Here's how the part is built. I have some questions about the finished solid (model axes, mm). Coordinates: 2 decimals unless noted, no trailing zeros. Write each loop counter-clockwise with the first axis right and the second up, starting at its lowest first coordinate (ties: lowest second). Pieces come first, ordered by that corner, then holes.
Item 1: If we section it at A-A (y = 0): Please give me the cut outline in (x, z).
Item 2: We'd pull the mould along Z, two halves only. Please class faces 1 (the face through (4.93, -9.902, -49.786)), 2 (the face through (5, 5, -42)), 3 (the face through (5, -57, -82)), 4 (the face through (4.93, -37.92, -66.82)): +Z half, -Z half, draft (parallel to the pull), parting line (faces both ways), or undercut.
Item 3: I'm going to push a flat-ended pin straight in: pin 1 Ø5 at (y, z) = (-9.58, -66.75) entering from +X. Where does the tip first touch, or does it pass through?
Item 4: If we section it at B-B (z = -23): Please give me the cut outline in (x, y), then the cut area to 3 significant figures.
Item 5: If we section it at C-C (z = -39): Please give me the cut outline in (x, y), then the cut area to 3 significant figures.
Item 6: If we section it at D-D (y = -16.5): Please give me the cut outline in (x, z).
Item 7: If I drill on line 1 (Z direction, x = 5.5, y = -23); line 2 (Y direction, x = 5, z = -66.75); line 3 (Z direction, x = 6.5, y = -30), over which ranges is the centre line in solid material (lowest first)?
Autodesk Inventor part; units mm, degrees
ref_plane "YZ Plane" through (0, 0, 0) normal (1, 0, 0) x (0, 1, 0)
ref_plane "XZ Plane" through (0, 0, 0) normal (0, 1, 0) x (-1, 0, 0)
ref_plane "XY Plane" through (0, 0, 0) normal (0, 0, 1) x (1, 0, 0)
sketch "Esquisse1" plane through (0, 0, 0) normal (1, 0, 0) x (0, 1, 0)
  line L0 (0, 0) -> (-126, 0)
  line L1 (-126, -82) -> (0, -82)
  circle A0 centre (-23, -23) radius 18
  circle A1 centre (-23, -59) radius 18
  circle A2 centre (-116.2792, -41) radius 4
  line L2 (-120.2792, 0) -> (-120.2792, -82)
  circle A3 centre (-30, -59) radius 6
  circle A4 centre (-23, -43.5) radius 1.5
  circle A5 centre (-23, -74.5) radius 1.5
  circle A6 centre (-9.5766, -51.25) radius 1.5
  circle A7 centre (-9.5766, -66.75) radius 1.5
  line L3 (-23, -59) -> (-30, -59)
  line L4 (-23, -59) -> (-23, -43.5)
  line L5 (-23, -59) -> (-23, -74.5)
  circle A8 centre (-36.4234, -51.25) radius 1.5
  circle A9 centre (-36.4234, -66.75) radius 1.5
  line L6 (0, -82) -> (5, -82)
  line L7 (5, -82) -> (5, 0)
  line L8 (5, 0) -> (0, 0)
  line L9 (-5, -82) -> (-5, 0)
  line L10 (0, -72) -> (0, -10)
  circle A10 centre (0, -72) radius 2
  circle A11 centre (0, -10) radius 2
  line L11 (5, 0) -> (0, 0)
  line L12 (5, -82) -> (-5, -82)
  line L13 (-107.2792, -10) -> (-107.2792, -72)
  circle A12 centre (-107.2792, -10) radius 2
  circle A13 centre (-107.2792, -72) radius 2
  line L14 (-120.2792, 0) -> (-126, 0)
  line L15 (-126, 0) -> (-126, -82)
  line L16 (-126, -82) -> (-120.2792, -82)
  line L17 (-120.2792, -82) -> (-120.2792, 0)
  dimension "d0" = 82
  dimension "d2" = 36
  dimension "d3" = 23
  dimension "d4" = 36
  dimension "d5" = 23
  dimension "d6" = 8
  dimension "d7" = 95
  dimension "d8" = 41
  dimension "d12" = 4
  dimension "d13" = 12
  dimension "d14" = 7
  dimension "d15" = 3
  dimension "d16" = 15.5
  dimension "d17" = 3
  dimension "d18" = 15.5
  dimension "d19" = 3
  dimension "d20" = 3
  dimension "d21" = 60
  dimension "d22" = 60
  dimension "d23" = 15.5
  dimension "d25" = 0
  dimension "d26" = 15.5
  dimension "d27" = 3
  dimension "d28" = 3
  dimension "d29" = 15.5
  dimension "d30" = 15.5
  dimension "d31" = 60
  dimension "d32" = 60
  dimension "d38" = 82
  dimension "d39" = 28
  dimension "d40" = 10
  dimension "d41" = 5
  dimension "d42" = 62
  dimension "d43" = 10
  dimension "d44" = 4
  dimension "d45" = 4
  dimension "d46" = 5
  dimension "d47" = 82
  dimension "d48" = 10
  dimension "d49" = 28
  dimension "d61" = 62
  dimension "d62" = 13
  dimension "d63" = 10
  dimension "d64" = 4
  dimension "d65" = 4
  dimension "d76" = 126
  dimension "d77" = 126
extrude "Extrusion1" add sketch "Esquisse1" along normal blind 10 contours L9 A0 A1 L1 L2 L0 | L9 A1 A0 | A1 | A13 | A12
sketch "Esquisse2" plane through (10, -23, -23) normal (1, 0, 0) x (0, 0, -1)
  line L0 (0, 18) -> (-23, 18)
  line L1 (-23, 18) -> (59, 18)
  line L2 (59, 18) -> (59, 28)
  line L3 (59, 28) -> (-23, 28)
  line L4 (-23, 28) -> (-23, 18)
  line L5 (-13, 23) -> (49, 23)
  circle A0 centre (-13, 23) radius 2
  circle A1 centre (49, 23) radius 2
  point P0 (-23, 23)
  dimension "d52" = 82
  dimension "d53" = 10
  dimension "d54" = 62
  dimension "d55" = 10
  dimension "d56" = 4
  dimension "d57" = 4
  dimension "d58" = 5
extrude "Extrusion2" add sketch "Esquisse2" against normal blind 10
sketch "Esquisse3" plane through (10, -116.2792, -41) normal (1, 0, 0) x (0, 0, -1)
  line L0 (-31, 9) -> (31, 9)
  line L1 (-41, 121.2792) -> (-41, -4)
  line L2 (-41, -4) -> (0, -4)
  point P0 (-41, 116.2792)
  dimension "d66" = 62
  dimension "d67" = 10
  dimension "d68" = 13
hole "Perçage1" at (10, -107.2792, -10) at (10, -107.2792, -72) direction (-1, 0, 0) diameter 4 end through all
sketch "Esquisse4" plane through (0, -120.2792, -41) normal (0, -1, 0) x (1, 0, 0)
  line L0 (0, 0) -> (0, -41)
  line L1 (10, 41) -> (0, 41)
  line L2 (0, 41) -> (0, -41)
  line L3 (0, -41) -> (10, -41)
  line L4 (10, -41) -> (10, 41)
  dimension "d78" = 10
  dimension "d79" = 82
extrude "Extrusion3" add sketch "Esquisse4" along normal blind 0.72
properties part number "paroismoteur"
Answer list:
1. outline: (0, -82) - (10, -82) - (10, -74) - (0, -74) - close; (0, -70) - (10, -70) - (10, -12) - (0, -12) - close; (0, -8) - (10, -8) - (10, 0) - (0, 0) - close
2. face 1: undercut
2. face 2: draft
2. face 3: -Z half
2. face 4: undercut
3. pin 1: stops at x = 10
4. outline: (0, -121) - (10, -121) - (10, -41) - (0, -41) - close; (0, -5) - (10, -5) - (10, 5) - (0, 5) - close
4. area: 900 mm2
5. outline: (0, -121) - (10, -121) - (10, -119.74) - (0, -119.74) - close; (0, -112.82) - (10, -112.82) - (10, -31.25) - (0, -31.25) - close; (0, -14.75) - (10, -14.75) - (10, 5) - (0, 5) - close
5. area: 1,030 mm2
6. outline: (0, -82) - (10, -82) - (10, -39.79) - (0, -39.79) - close; (0, -6.21) - (10, -6.21) - (10, 0) - (0, 0) - close
7. line 1: z = -82 to -76, -73 to -45, -42 to -41, -5 to 0
7. line 2: y = -121 to -37.92, -34.92 to -11.08, -8.08 to 5
7. line 3: z = -82 to -65, -53 to -39.58, -6.42 to 0
